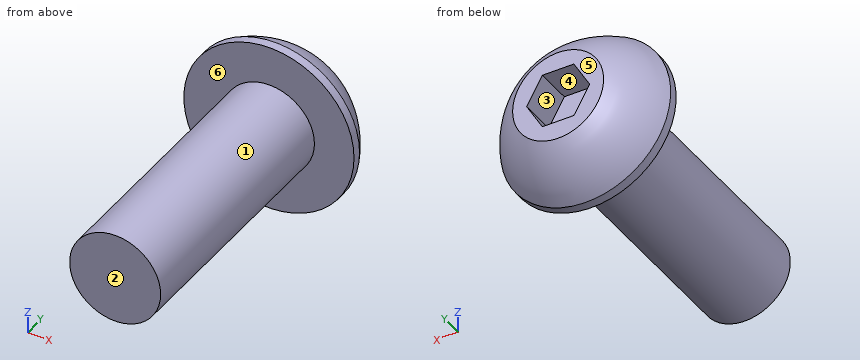
```python
from build123d import *

# Parameters (mm, degrees)
CUT_EXTRUDE1_DEPTH = 2


with BuildPart() as part:
    # Sketch1 → Revolve1 (revolve)
    with BuildSketch(Plane.XY):
        with BuildLine():
            Line((2.5, 0), (4.675, 0))
            Line((4.675, 0), (4.675, 0.5))
            ThreePointArc((4.675, 0.5), (3.763510598, 1.90312922), (2.5, 3))
            Line((2.5, 3), (0, 3))
            Line((0, 3), (0, -14))
            Line((0, -14), (2.5, -14))
            Line((2.5, -14), (2.5, 0))
        make_face()
    revolve(axis=Axis((0, -14, 0), (0, 1, 0)))

    # Sketch2 → Cut-Extrude1 (cut)
    with BuildSketch(Plane(origin=(0, 3, 0), x_dir=(1, 0, 0), z_dir=(0, 1, 0))):
        Polygon((0.866025404, 1.5), (-0.866025404, 1.5), (-1.732050808, 0), (-0.866025404, -1.5), (0.866025404, -1.5), (1.732050808, 0), align=None)
    extrude(amount=-CUT_EXTRUDE1_DEPTH, mode=Mode.SUBTRACT)


solid = part.part
```
Verification items for the finished model (mm, model axes). Face numbers are marked on the shaded views. A direction names the side the tool comes from. Round coordinates to 2 decimals unless told otherwise and drop trailing zeros. Write each loop counter-clockwise with the first axis right and the second up, starting at its lowest first coordinate (ties: lowest second). Pieces come first, ordered by that corner, then holes. Notation, with made-up numbers: (33, 53) - (43, 53) arc R16 cw to (43, 75) - close; hole circle Ø3 at (29, 1). An arc over 180 degrees is marked (long way). Answer as a JSON object with one key per item and string values. Group by question number.
Q1. Mould release check, pull along Z, two halves, no side actions. Record for the marked faces 1, 2 and 3: released by +Z, released by -Z, zero draft, split by the parting line, or undercut.
Q2. Thickness scan on line 1 (Y direction, x = -2.5, z = 3); line 2 (X direction, y = -1.25, z = 0); line 3 (Y direction, x = -0.25, z = 0). Record the ranges inside material, lowest first.
Q3. Go/stop test with flat-tipped pins: pin 1 Ø3 at (y, z) = (-8, 1.5) entering from +X; pin 2 Ø0.5 at (x, y) = (-0.5, 2.5) entering from +Z; pin 3 Ø1.4 at (x, y) = (0, 2) entering from -Z; pin 4 Ø1.5 at (y, z) = (-9, 3.5) entering from +X. Record where each tip stops, or that it passes through.
Q4. Section check A-A, the plane y = -3.25. Enter the section's corners in (x, z).
Q5. Tool access check on the marked faces 4, 5 and 6. Record the directions out of +Z, -Z, +X, -X, +Y, -Y that give a thin tool (end or side, any length) a straight path to the whole face; none if there is none.
Found:
{
 "1": {"face 1": "split by the parting line", "face 2": "zero draft", "face 3": "undercut"},
 "2": {"line 1": "y = 0 to 1.73", "line 2": "x = -2.5 to 2.5", "line 3": "y = -14 to 1"},
 "3": {"pin 1": "stops at x = 2.5", "pin 2": "stops at z = 3.4", "pin 3": "stops at z = -4.22", "pin 4": "passes through"},
 "4": {"outline": "circle Ø5 at (0, 0)"},
 "5": {"face 4": "+Y", "face 5": "+Z, -Z, +X, -X, +Y", "face 6": "-Y"}
}
